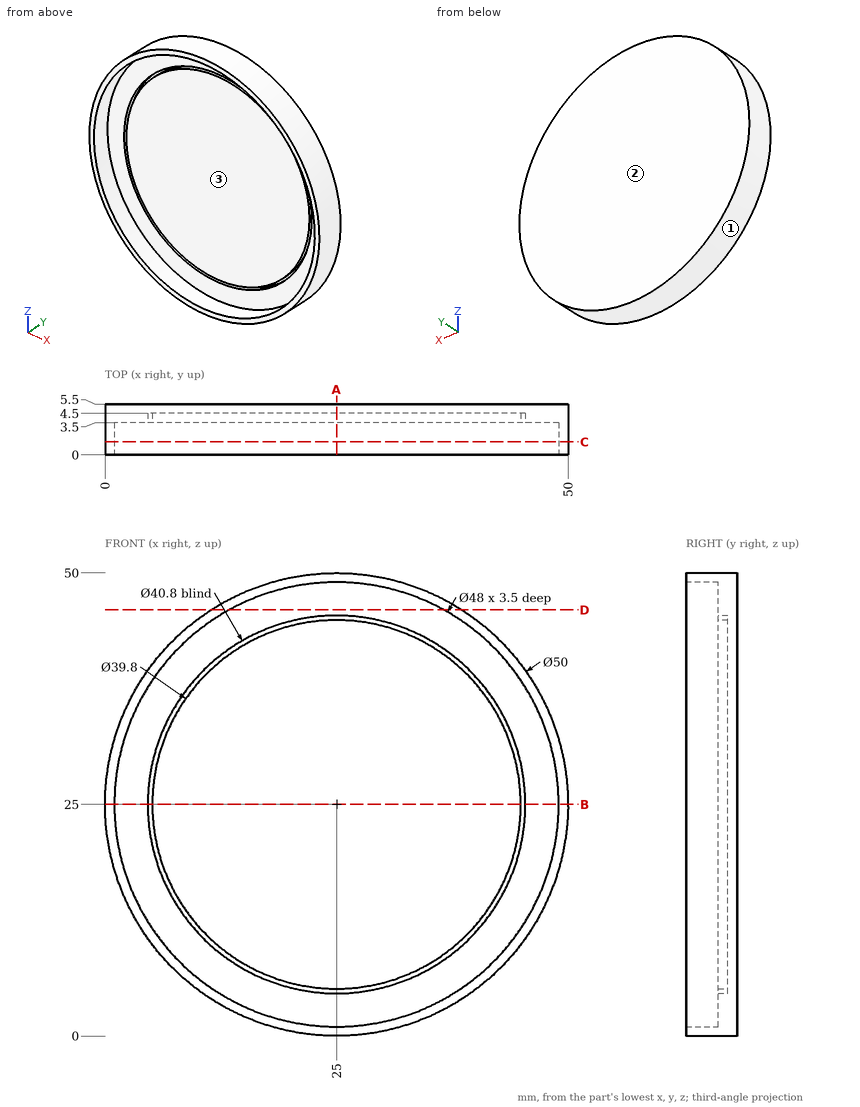
The figure shows three views and two pictorial views of one solid part (mm, origin at its lowest corner). Answer the questions. Round coordinates to 2 decimals unless told otherwise and drop trailing zeros. Write each loop counter-clockwise with the first axis right and the second up, starting at its lowest first coordinate (ties: lowest second). Pieces come first, ordered by that corner, then holes. Notation, with made-up numbers: (-8, 64) - (44, 64) arc R16 ccw to (44, 89) - close; hole circle Ø8 at (19, -40). An arc over 180 degrees is marked (long way). Answer in a Markdown table with one row per item. Add a question column.
1. A cutting plane is placed at D-D, the plane z = 46. Determine the outline of the cut face in (x, y).
2. Given pin 1 (20 mm diameter, centred on x = 21.5, z = 25.5, fed in from -Y); pin 2 (1 mm diameter, centred on y = 2, z = 8.5, fed in from +X); pin 3 (1.5 mm diameter, centred on y = 2.5, z = 23, fed in from +X), each flat-ended and moving along its own axis, determine where each tip first touches the part or whether it passes through.
3. A cutting plane is placed at C-C, the plane y = 1.4. Determine the outline of the cut face in (x, z).
4. The mould has two halves that part along Z. Classify the marked faces 1, 2 and 3: +Z half, -Z half, draft (parallel to the pull), parting line (faces both ways), or undercut.
5. A cutting plane is placed at B-B, the plane z = 25. Determine the outline of the cut face in (x, y).
6. A cutting plane is placed at A-A, the plane x = 25. Determine the outline of the cut face in (y, z), and give its area (3 significant figures).
7. Find the intervals of material crossed by line 1 along X through (y, z) = (4.25, 25); line 2 along X through (y, z) = (3.9, 29); line 3 along Y through (x, z) = (29, 31), in increasing order. Write a range as from..to.
Worked out:
| question | item | result |
|---|---|---|
| 1 | outline | (11.44, 0) - (13.38, 0) - (13.38, 3.5) - (36.62, 3.5) - (36.62, 0) - (38.56, 0) - (38.56, 5.5) - (11.44, 5.5) - close |
| 2 | pin 1 | y = 3.5 |
| 2 | pin 2 | x = 44.21 |
| 2 | pin 3 | x = 49.97 |
| 3 | outline | circle Ø50 at (25, 25); hole circle Ø48 at (25, 25) |
| 4 | face 1 | parting line |
| 4 | face 2 | draft |
| 4 | face 3 | undercut |
| 5 | outline | (0, 0) - (1, 0) - (1, 3.5) - (4.6, 3.5) - (4.6, 4.5) - (5.1, 4.5) - (5.1, 3.5) - (44.9, 3.5) - (44.9, 4.5) - (45.4, 4.5) - (45.4, 3.5) - (49, 3.5) - (49, 0) - (50, 0) - (50, 5.5) - (0, 5.5) - close |
| 6 | outline | (0, 0) - (5.5, 0) - (5.5, 50) - (0, 50) - (0, 49) - (3.5, 49) - (3.5, 45.4) - (4.5, 45.4) - (4.5, 44.9) - (3.5, 44.9) - (3.5, 5.1) - (4.5, 5.1) - (4.5, 4.6) - (3.5, 4.6) - (3.5, 1) - (0, 1) - close |
| 6 | area | 106 mm^2 |
| 7 | line 1 | 0..4.6, 5.1..44.9, 45.4..50 |
| 7 | line 2 | 0.32..5, 5.51..44.49, 45..49.68 |
| 7 | line 3 | 3.5..5.5 |
